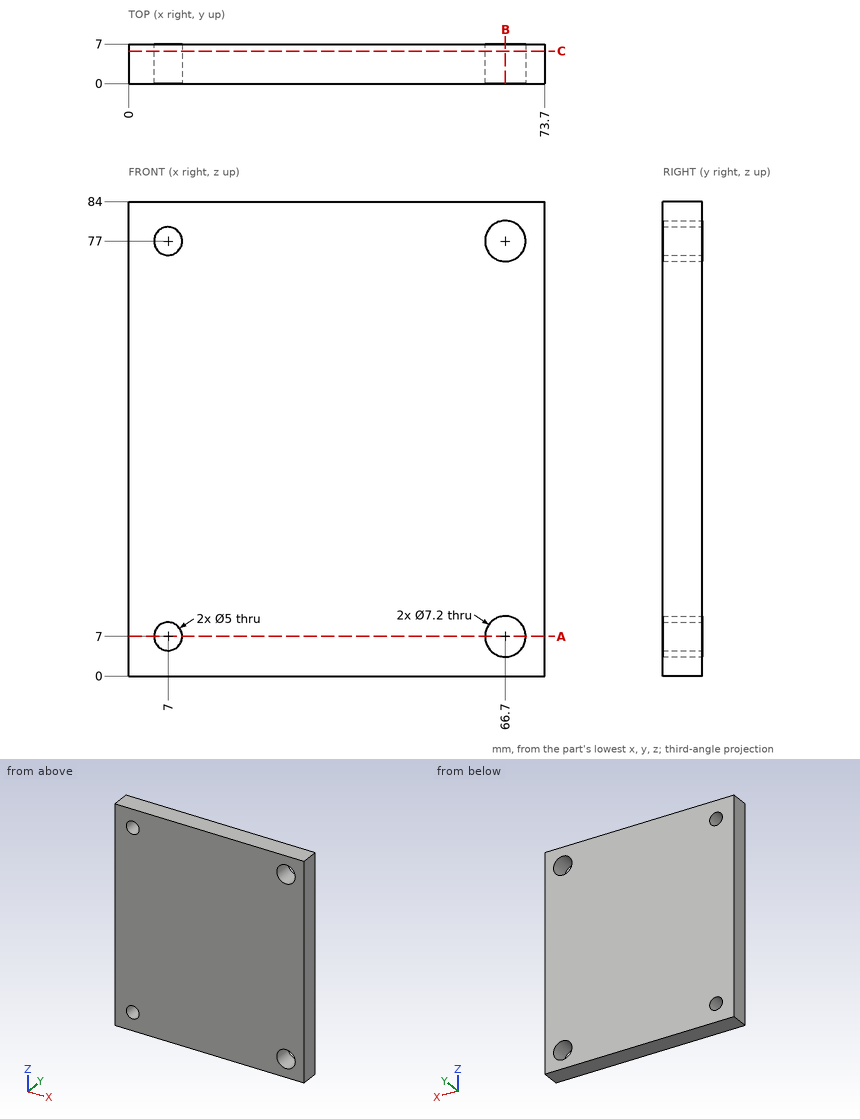
Geometry check sheet. Reference: drawing and pictorial views, mm from the part's lowest x, y, z. Round coordinates to 2 decimals unless told otherwise and drop trailing zeros. Order: outer loops, then holes, each group sorted by start corner. A loop starts at its lowest first (then second) coordinate and runs counter-clockwise, first axis right, second up.
Q1. Cross-section at A-A, the plane z = 7. Enter the section's corners in (x, y).
Filled sheet:
outline: (0, 0) - (4.5, 0) - (4.5, 7) - (0, 7) - close; (9.5, 0) - (63.1, 0) - (63.1, 7) - (9.5, 7) - close; (70.3, 0) - (73.7, 0) - (73.7, 7) - (70.3, 7) - close
Q2. Depth check by flat-ended pin: P1, Ø8.5, axis at x = 66.7, z = 77, coming from the +Y side. Enter the tip coordinate at first touch or a pass-through.
Filled sheet:
P1: stops at y = 7
Q3. Cross-section at C-C, the plane y = 5.75. Enter the section's corners in (x, z), plus the area to 3 significant figures.
Filled sheet:
outline: (0, 0) - (73.7, 0) - (73.7, 84) - (0, 84) - close; hole circle Ø5 at (7, 7); hole circle Ø5 at (7, 77); hole circle Ø7.2 at (66.7, 7); hole circle Ø7.2 at (66.7, 77)
area: 6,070 mm2
Q4. Cross-section at B-B, the plane x = 66.7. Enter the section's corners in (y, z), plus the area to 3 significant figures.
Filled sheet:
outline: (0, 0) - (7, 0) - (7, 3.4) - (0, 3.4) - close; (0, 10.6) - (7, 10.6) - (7, 73.4) - (0, 73.4) - close; (0, 80.6) - (7, 80.6) - (7, 84) - (0, 84) - close
area: 487 mm2
Q5. Scan lines: L1, parallel to Z at x = 7, y = 2; L2, parallel to Z at x = 66.7, y = 4.5; L3, parallel to X at y = 5.5, z = 6. Record each from-to range of solid material in increasing order.
Filled sheet:
L1: z = 0 to 4.5, 9.5 to 74.5, 79.5 to 84
L2: z = 0 to 3.4, 10.6 to 73.4, 80.6 to 84
L3: x = 0 to 4.71, 9.29 to 63.24, 70.16 to 73.7
